from build123d import *

# Parameters (mm, degrees)
F0_R     = 4.725
F1_DEPTH = 3.25


with BuildPart() as f1:
    # F0 (on Top) → F1 (new body, symmetric)
    with BuildSketch(Plane.XY):
        with BuildLine():
            Line((-16.5, -12.7), (16.5, -12.7))
            ThreePointArc((16.5, -12.7), (18.267767, -11.967767), (19, -10.2))
            Line((19, -10.2), (19, 10.2))
            ThreePointArc((19, 10.2), (18.267767, 11.967767), (16.5, 12.7))
            Line((16.5, 12.7), (-16.5, 12.7))
            ThreePointArc((-16.5, 12.7), (-18.267767, 11.967767), (-19, 10.2))
            Line((-19, 10.2), (-19, -10.2))
            ThreePointArc((-19, -10.2), (-18.267767, -11.967767), (-16.5, -12.7))
        make_face()
        with Locations((-8, 0)):
            Circle(F0_R, mode=Mode.SUBTRACT)
        with BuildLine():
            ThreePointArc((12.725, 0), (8, -4.725), (3.275, 0))
            ThreePointArc((3.275, 0), (8, 4.725), (12.725, 0))
        make_face(mode=Mode.SUBTRACT)
    extrude(amount=F1_DEPTH, both=True)


solid = f1.part
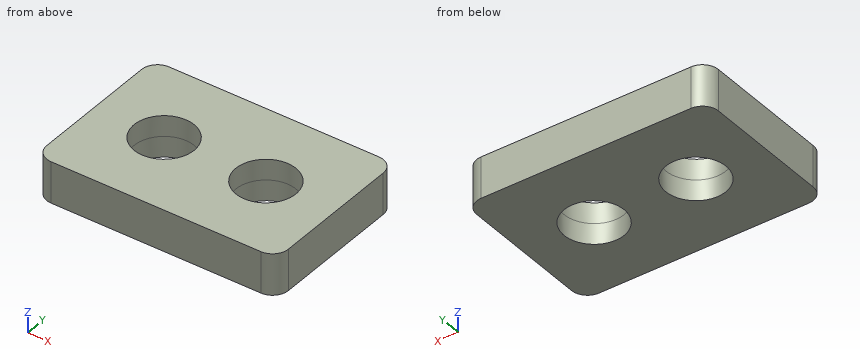
Source: CAD feature listing. Evaluate the final solid. Frame: model axes, mm. Coordinates: 2 decimals unless noted, no trailing zeros. Loops run counter-clockwise (first coordinate to the right, second up) from the corner with the lowest first, then second, coordinate; pieces in that order, holes last. Notation, with made-up numbers: M 47.5,-38.75 L 71.5,-38.75 A16 cw 71.5,-20.75 Z; hole C 43.25,5 d10. An arc over 180 degrees is marked long. Answer in a Markdown table with one row per item.
Q1. Section D-D on x = 10.5. Return the cut outline in (y, z), plus the area to 3 significant figures.
Answers below:
| item | result |
|---|---|
| outline | M -12.7,-3.25 L -4.01,-3.25 L -4.01,3.25 L -12.7,3.25 Z; M 4.01,-3.25 L 12.7,-3.25 L 12.7,3.25 L 4.01,3.25 Z |
| area | 113 mm^2 |
Q2. Section C-C on z = 0.5. Return the cut outline in (x, y) (3 decimals), plus the area to 3 significant figures.
Answers below:
| item | result |
|---|---|
| outline | M -19,-10.2 A2.5 ccw -16.5,-12.7 L 16.5,-12.7 A2.5 ccw 19,-10.2 L 19,10.2 A2.5 ccw 16.5,12.7 L -16.5,12.7 A2.5 ccw -19,10.2 Z; hole C -8,0 d9.45; hole C 8,0 d9.45 |
| area | 820 mm^2 |
Q3. Ray query, probe 1 along Y at (x, z) = (8, -1.35) (3 decimals); probe 2 along X at (y, z) = (-0.75, 0.5); probe 3 along X at (y, z) = (-4, 3). Return the intervals inside material, ascending. Write a range as from..to.
Answers below:
| item | result |
|---|---|
| probe 1 | y = -12.7..-4.725, 4.725..12.7 |
| probe 2 | x = -19..-12.67, -3.33..3.33, 12.67..19 |
| probe 3 | x = -19..-10.52, -5.48..5.48, 10.52..19 |
Q4. Section B-B on y = 0. Return the cut outline in (x, z) (3 decimals).
Answers below:
| item | result |
|---|---|
| outline | M -19,-3.25 L -12.725,-3.25 L -12.725,3.25 L -19,3.25 Z; M -3.275,-3.25 L 3.275,-3.25 L 3.275,3.25 L -3.275,3.25 Z; M 12.725,-3.25 L 19,-3.25 L 19,3.25 L 12.725,3.25 Z |
Q5. Section A-A on x = -8. Return the cut outline in (y, z) (3 decimals), plus the area to 3 significant figures.
Answers below:
| item | result |
|---|---|
| outline | M -12.7,-3.25 L -4.725,-3.25 L -4.725,3.25 L -12.7,3.25 Z; M 4.725,-3.25 L 12.7,-3.25 L 12.7,3.25 L 4.725,3.25 Z |
| area | 104 mm^2 |
